Verification items for this drawing (mm, ordinates from the low corner). A direction names the side the tool comes from. Round coordinates to 2 decimals unless told otherwise and drop trailing zeros. Order: outer loops, then holes, each group sorted by start corner. A loop starts at its lowest first (then second) coordinate and runs counter-clockwise, first axis right, second up.
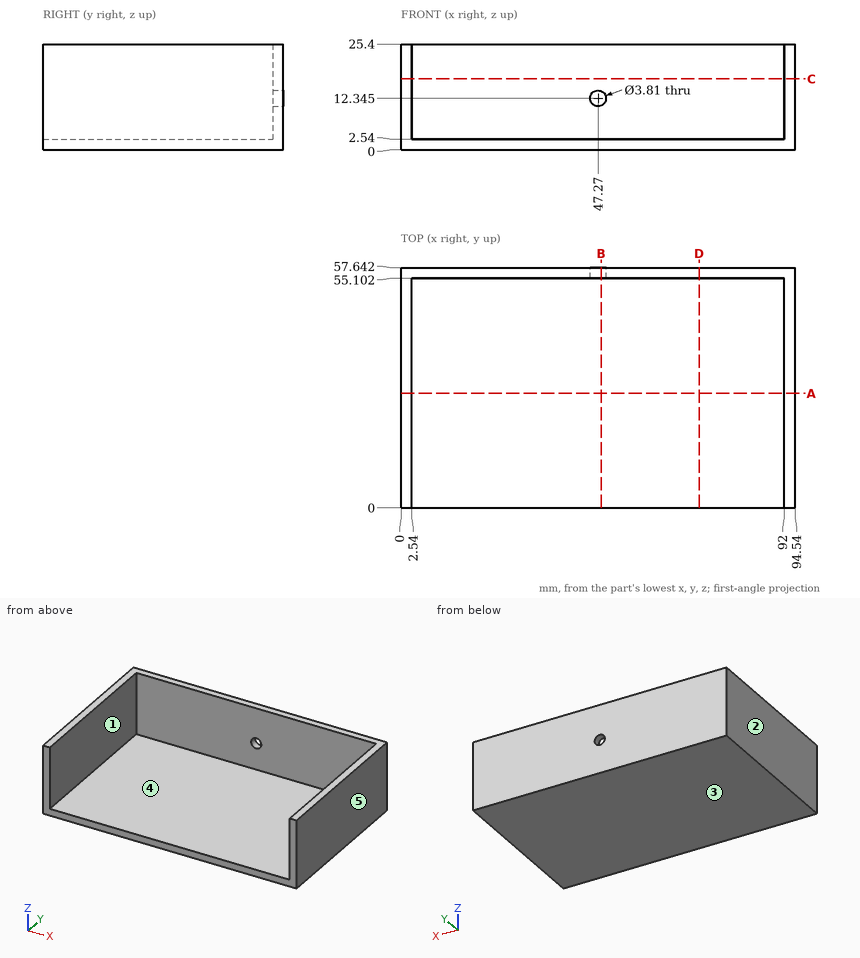
Item 1: Sectioned sample at B-B (x = 48). Record the cut outline in (y, z) (1 decimal).
Answer:
outline: (0, 0) - (57.6, 0) - (57.6, 10.6) - (55.1, 10.6) - (55.1, 2.5) - (0, 2.5) - close; (55.1, 14.1) - (57.6, 14.1) - (57.6, 25.4) - (55.1, 25.4) - close
Item 2: Scan lines: line 1 along X through (y, z) = (41, 22.25); line 2 along Y through (x, z) = (89, 19.25); line 3 along Z through (x, y) = (39, 25). Record each from-to range of solid material in increasing order.
Answer:
line 1: x = 0 to 2.54, 92 to 94.54
line 2: y = 55.1 to 57.64
line 3: z = 0 to 2.54
Item 3: Sectioned sample at D-D (x = 71.5). Record the cut outline in (y, z).
Answer:
outline: (0, 0) - (57.64, 0) - (57.64, 25.4) - (55.1, 25.4) - (55.1, 2.54) - (0, 2.54) - close
Item 4: Release check for a two-part mould opening along X. For the marked faces 1, 2 and 3 record: released by +X, released by -X, zero draft, split by the parting line, or undercut.
Answer:
face 1: undercut
face 2: released by -X
face 3: zero draft
Item 5: Go/stop test with flat-tipped pins: P1, Ø6, axis at x = 56, z = 18, coming from the -Y side; P2, Ø16.5, axis at x = 66, y = 33.5, coming from the +Z side; P3, Ø2.5, axis at x = 47.27, z = 12.35, coming from the -Y side. Record where each tip stops, or that it passes through.
Answer:
P1: stops at y = 55.1
P2: stops at z = 2.54
P3: passes through
Item 6: Access from +Z, -Z, +X, -X, +Y, -Y to the whole of each face (thin tool, end or side, straight path). Record for the marked faces 4 and 5.
Answer:
face 4: +Z, -Y
face 5: +Z, -Z, +X, +Y, -Y
Item 7: Sectioned sample at A-A (y = 27.5). Record the cut outline in (x, z).
Answer:
outline: (0, 0) - (94.54, 0) - (94.54, 25.4) - (92, 25.4) - (92, 2.54) - (2.54, 2.54) - (2.54, 25.4) - (0, 25.4) - close
Item 8: Sectioned sample at C-C (z = 17). Record the cut outline in (x, y).
Answer:
outline: (0, 0) - (2.54, 0) - (2.54, 55.1) - (92, 55.1) - (92, 0) - (94.54, 0) - (94.54, 57.64) - (0, 57.64) - close
